Verification items for the finished model (mm, model axes). Give positions to 0.01 mm unless a question says otherwise; leave off trailing zeros. Order: outer loops, then holes, each group sorted by start corner. A loop starts at its lowest first (then second) coordinate and runs counter-clockwise, first axis right, second up. Notation, with made-up numbers: (-24, 54.5) -> (22, 54.5) arc R29 cw to (22, 90.5) -> close; hole circle Ø5 at (30.5, 50). An arc over 180 degrees is marked (long way). Return JSON: item names as keys, results as strings. Group by question number.
(1) Thickness scan on line 1 along X through (y, z) = (380.5, -21.5); line 2 along X through (y, z) = (342, -271); line 3 along X through (y, z) = (81, -193). Record the ranges inside material, lowest first.
(2) Cross-section at C-C on x = -60.5. Enter the section's corners in (y, z).
(3) Cross-section at B-B on z = -30. Enter the section's corners in (x, y).
(4) Release check for a two-part mould opening along X. For faces 1 (the face through (-68.659, 246.5, -278.065)), 2 (the face through (30, 246, -36)), 3 (the face through (31.15, 246, -39)) record: pulls with the +X half, pulls with the -X half, needs draft (parallel to the pull), parting line crosses it, or undercut.
(5) Depth check by flat-ended pin: pin 1 Ø8 at (x, y) = (-191, 288) entering from -Z; pin 2 Ø5 at (x, y) = (-47.5, 397) entering from -Z; pin 3 Ø10 at (y, z) = (306, -141) entering from +X. Enter the tip coordinate at first touch or a pass-through.
(6) Cross-section at A-A on y = 281. Enter the section's corners in (x, z), then the cut area to 3 significant figures.
from build123d import *

# Parameters (mm, degrees)
SALIENTE_EXTRUIR1_DEPTH = 500


with BuildPart() as part:
    # Croquis3 → Saliente-Extruir1 (new body)
    with BuildSketch(Plane(origin=(0, 0, 0), x_dir=(1, 0, 0), z_dir=(0, 1, 0))):
        with BuildLine():
            Line((31.15, 127.741818938), (31.15, -52.258181062))
            Line((31.15, -52.258181062), (30, -52.258181062))
            Line((30, -52.258181062), (30, 127.741818938))
            ThreePointArc((30, 127.741818938), (-71.147319607, 279.11948034), (-249.709446097, 243.601265035))
            Line((-249.709446097, 243.601265035), (-250.522618896, 244.414437834))
            ThreePointArc((-250.522618896, 244.414437834), (-70.70723366, 280.181941802), (31.15, 127.741818938))
        make_face()
    extrude(amount=SALIENTE_EXTRUIR1_DEPTH)


solid = part.part
Verdict:
{
 "1": {"line 1": "30 to 31.15", "line 2": "-215.72 to -213.37, -54.33 to -51.98", "line 3": "16.44 to 17.7"},
 "2": {"outline": "(0, -275.54) -> (500, -275.54) -> (500, -274.26) -> (0, -274.26) -> close"},
 "3": {"outline": "(30, 0) -> (31.15, 0) -> (31.15, 500) -> (30, 500) -> close"},
 "4": {"face 1": "undercut", "face 2": "pulls with the -X half", "face 3": "pulls with the +X half"},
 "5": {"pin 1": "z = -283.95", "pin 2": "z = -269.85", "pin 3": "x = 30.94"},
 "6": {"outline": "(-250.52, -244.41) arc R165 ccw to (31.15, -127.74) -> (31.15, 52.26) -> (30, 52.26) -> (30, -127.74) arc R163.85 cw to (-249.71, -243.6) -> close", "area": "653 mm²"}
}
